Here's how the part is built. I have some questions about the finished solid (model axes, mm). Face numbers are marked on the shaded views. A direction names the side the tool comes from. Give positions to 0.01 mm unless a question says otherwise; leave off trailing zeros. Loops run counter-clockwise (first coordinate to the right, second up) from the corner with the lowest first, then second, coordinate; pieces in that order, holes last.
Q1. If we section it at A-A (y = 7): Please give me the cut outline in (x, z).
Q2. Will these pins go through, and if not, where does the flat tip stop? P1, Ø2, axis at x = -23.5, y = 5, coming from the +Z side; P2, Ø5, axis at y = 3.5, z = 8, coming from the +X side; P3, Ø5, axis at y = 4, z = 21, coming from the +X side; P4, Ø2, axis at x = 14, z = -3, coming from the +Y side.
Q3. If we section it at D-D (x = -5.5): Please give me the cut outline in (y, z).
Q4. I need wall thicknesses on line 1 (X direction, y = -4.25, z = 23); line 2 (Y direction, x = -2, z = -4); line 3 (X direction, y = -5, z = 13). Which ranges of each line are inside material? Lowest first, please.
Q5. We'd pull the mould along X, two halves only. Please class the marked faces 1, 2 and 3: +X half, -X half, draft (parallel to the pull), parting line (faces both ways), or undercut.
Q6. If we section it at C-C (z = -1): Please give me the cut outline in (x, y), plus the area to 3 significant figures.
Q7. If we section it at B-B (y = -3.5): Please give me the cut outline in (x, z), plus the area to 3 significant figures.
Q8. For the marked faces 4 and 5, which set-ups out of +Z, -Z, +X, -X, +Y, -Y let a thin tool reach every point of the face, with its end or its side?
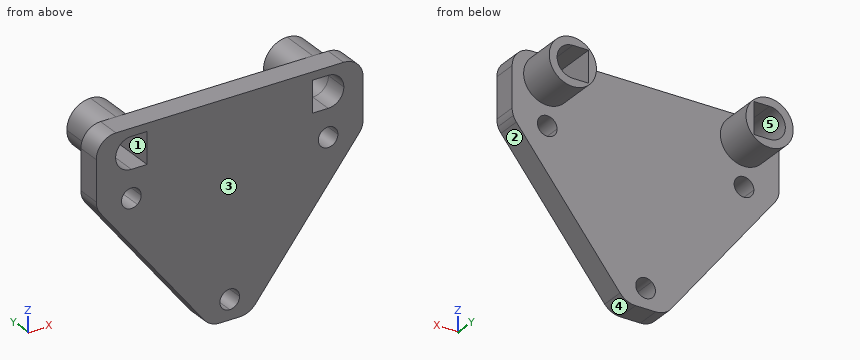
from build123d import *

# Parameters (mm, degrees)
F1_DEPTH = 6
F3_DEPTH = 10


with BuildPart() as f1:
    # F0 (on Front) → F1 (new body)
    with BuildSketch(Plane.XZ):
        with BuildLine():
            Line((-22.5, 14.5380757153), (-15.95, 14.5380757153))
            Line((-15.95, 14.5380757153), (15.95, 14.5380757153))
            Line((15.95, 14.5380757153), (22.5, 14.5380757153))
            ThreePointArc((22.5, 14.5380757153), (25, 17.0380757153), (27.5, 14.5380757153))
            Line((27.5, 14.5380757153), (33.6112053721, 14.5380757153))
            ThreePointArc((33.6112053721, 14.5380757153), (33.8410734014, 15.3874164322), (33.9184952978, 16.2639007813))
            Line((33.9184952978, 16.2639007813), (33.9184952978, 19.5380757153))
            Line((33.9184952978, 19.5380757153), (25, 19.5380757153))
            Line((25, 19.5380757153), (-25, 19.5380757153))
            Line((-25, 19.5380757153), (-33.9184952978, 19.5380757153))
            Line((-33.9184952978, 19.5380757153), (-33.9184952978, 16.2639007813))
            ThreePointArc((-33.9184952978, 16.2639007813), (-33.8410734014, 15.3874164322), (-33.6112053721, 14.5380757153))
            Line((-33.6112053721, 14.5380757153), (-27.5, 14.5380757153))
            ThreePointArc((-27.5, 14.5380757153), (-25, 17.0380757153), (-22.5, 14.5380757153))
        make_face()
        with BuildLine():
            Line((15.95, 14.5380757153), (-15.95, 14.5380757153))
            Line((-15.95, 14.5380757153), (-22.5, 14.5380757153))
            ThreePointArc((-22.5, 14.5380757153), (-22.7521952698, 13.4438299043), (-23.457899116, 12.5703549873))
            Line((-23.457899116, 12.5703549873), (-1.542100884, -15.3942035567))
            ThreePointArc((-1.542100884, -15.3942035567), (0, -14.8619242847), (1.542100884, -15.3942035567))
            Line((1.542100884, -15.3942035567), (23.457899116, 12.5703549873))
            ThreePointArc((23.457899116, 12.5703549873), (22.7521952698, 13.4438299043), (22.5, 14.5380757153))
            Line((22.5, 14.5380757153), (15.95, 14.5380757153))
        make_face()
        with BuildLine():
            ThreePointArc((-23.457899116, 12.5703549873), (-26.094245811, 12.2902709851), (-27.5, 14.5380757153))
            Line((-27.5, 14.5380757153), (-33.6112053721, 14.5380757153))
            ThreePointArc((-33.6112053721, 14.5380757153), (-33.28570797, 13.8292645711), (-32.8539367538, 13.1796990132))
            Line((-32.8539367538, 13.1796990132), (-6.5014092727, -20.4461260528))
            ThreePointArc((-6.5014092727, -20.4461260528), (-4.7544594387, -21.8575337451), (-2.5659678166, -22.3619242847))
            Line((-2.5659678166, -22.3619242847), (0, -22.3619242847))
            Line((0, -22.3619242847), (0, -19.8619242847))
            ThreePointArc((0, -19.8619242847), (-2.3631866008, -18.1776136189), (-1.542100884, -15.3942035567))
            Line((-1.542100884, -15.3942035567), (-23.457899116, 12.5703549873))
        make_face()
        with BuildLine():
            Line((33.6112053721, 14.5380757153), (27.5, 14.5380757153))
            ThreePointArc((27.5, 14.5380757153), (26.094245811, 12.2902709851), (23.457899116, 12.5703549873))
            Line((23.457899116, 12.5703549873), (1.542100884, -15.3942035567))
            ThreePointArc((1.542100884, -15.3942035567), (2.2478047302, -16.2676784737), (2.5, -17.3619242847))
            ThreePointArc((2.5, -17.3619242847), (1.767766953, -19.1296912377), (0, -19.8619242847))
            Line((0, -19.8619242847), (0, -22.3619242847))
            Line((0, -22.3619242847), (2.5659678166, -22.3619242847))
            ThreePointArc((2.5659678166, -22.3619242847), (4.7544594387, -21.8575337451), (6.5014092727, -20.4461260528))
            Line((6.5014092727, -20.4461260528), (32.8539367538, 13.1796990132))
            ThreePointArc((32.8539367538, 13.1796990132), (33.28570797, 13.8292645711), (33.6112053721, 14.5380757153))
        make_face()
        with BuildLine():
            Line((-33.9184952978, 26.5380757153), (-33.9184952978, 19.5380757153))
            Line((-33.9184952978, 19.5380757153), (-25, 19.5380757153))
            Line((-25, 19.5380757153), (-25, 21.5380757153))
            ThreePointArc((-25, 21.5380757153), (-29, 25.5380757153), (-25, 29.5380757153))
            Line((-25, 29.5380757153), (-25, 31.5380757153))
            Line((-25, 31.5380757153), (-28.9184952978, 31.5380757153))
            ThreePointArc((-28.9184952978, 31.5380757153), (-32.4540292037, 30.0736096212), (-33.9184952978, 26.5380757153))
        make_face()
        with BuildLine():
            Line((25, 19.5380757153), (33.9184952978, 19.5380757153))
            Line((33.9184952978, 19.5380757153), (33.9184952978, 26.5380757153))
            ThreePointArc((33.9184952978, 26.5380757153), (32.4540292037, 30.0736096212), (28.9184952978, 31.5380757153))
            Line((28.9184952978, 31.5380757153), (25, 31.5380757153))
            Line((25, 31.5380757153), (25, 29.5380757153))
            ThreePointArc((25, 29.5380757153), (27.8284271247, 28.36650284), (29, 25.5380757153))
            ThreePointArc((29, 25.5380757153), (27.8284271247, 22.7096485906), (25, 21.5380757153))
            Line((25, 21.5380757153), (25, 19.5380757153))
        make_face()
        Polygon((-25, 21.5380757153), (-25, 19.5380757153), (25, 19.5380757153), (25, 21.5380757153), (21, 21.5380757153), (21, 25.5380757153), (21, 29.5380757153), (25, 29.5380757153), (25, 31.5380757153), (-25, 31.5380757153), (-25, 29.5380757153), (-21, 29.5380757153), (-21, 25.5380757153), (-21, 21.5380757153), align=None)
    extrude(amount=F1_DEPTH)

    # F2 (on face) → F3 (join)
    with BuildSketch(Plane(origin=(0, 0, 0), x_dir=(-1, 0, 0), z_dir=(0, 1, 0))):
        with BuildLine():
            ThreePointArc((-25, 31.5380757153), (-29.2426406871, 21.2954350282), (-19, 25.5380757153))
            ThreePointArc((-19, 25.5380757153), (-20.7573593129, 29.7807164024), (-25, 31.5380757153))
        make_face()
        with BuildLine():
            Line((-21, 29.5380757153), (-21, 21.5380757153))
            Line((-21, 21.5380757153), (-25, 21.5380757153))
            ThreePointArc((-25, 21.5380757153), (-29, 25.5380757153), (-25, 29.5380757153))
            Line((-25, 29.5380757153), (-21, 29.5380757153))
        make_face(mode=Mode.SUBTRACT)
        with BuildLine():
            ThreePointArc((31, 25.5380757153), (29.2426406871, 29.7807164024), (25, 31.5380757153))
            ThreePointArc((25, 31.5380757153), (20.7573593129, 21.2954350282), (31, 25.5380757153))
        make_face()
        with BuildLine():
            Line((21, 29.5380757153), (25, 29.5380757153))
            ThreePointArc((25, 29.5380757153), (29, 25.5380757153), (25, 21.5380757153))
            Line((25, 21.5380757153), (21, 21.5380757153))
            Line((21, 21.5380757153), (21, 29.5380757153))
        make_face(mode=Mode.SUBTRACT)
    extrude(amount=F3_DEPTH)


solid = f1.part
Check sheet entries:
1. outline: circle Ø12 at (-25, 25.54); circle Ø12 at (25, 25.54); hole (-25, 21.54) - (-21, 21.54) - (-21, 29.54) - (-25, 29.54) arc R4 ccw to start; hole (21, 21.54) - (25, 21.54) arc R4 ccw to (25, 29.54) - (21, 29.54) - close
2. P1: stops at z = 31.52
2. P2: passes through
2. P3: stops at x = 30.64
2. P4: stops at y = 0
3. outline: (-6, -21.41) - (0, -21.41) - (0, 31.54) - (-6, 31.54) - close
4. line 1: x = -33.92 to -28.09, -21 to 21, 28.09 to 33.92
4. line 2: y = -6 to 0
4. line 3: x = -32.71 to -26.97, -23.03 to 23.03, 26.97 to 32.71
5. face 1: undercut
5. face 2: +X half
5. face 3: draft
6. outline: (-21.74, -6) - (21.74, -6) - (21.74, 0) - (-21.74, 0) - close
6. area: 261 mm2
7. outline: (-33.92, 16.26) arc R5 ccw to (-32.85, 13.18) - (-6.5, -20.45) arc R5 ccw to (-2.57, -22.36) - (2.57, -22.36) arc R5 ccw to (6.5, -20.45) - (32.85, 13.18) arc R5 ccw to (33.92, 16.26) - (33.92, 26.54) arc R5 ccw to (28.92, 31.54) - (-28.92, 31.54) arc R5 ccw to (-33.92, 26.54) - close; hole circle Ø5 at (-25, 14.54); hole (-25, 21.54) - (-21, 21.54) - (-21, 29.54) - (-25, 29.54) arc R4 ccw to start; hole circle Ø5 at (0, -17.36); hole (21, 21.54) - (25, 21.54) arc R4 ccw to (25, 29.54) - (21, 29.54) - close; hole circle Ø5 at (25, 14.54)
7. area: 2,400 mm2
8. face 4: -Z, +X, +Y, -Y
8. face 5: +Y, -Y
